The listing builds one solid part. Answer for the finished solid, in the listing's coordinates (mm). Face numbers are marked on the shaded views. A direction names the side the tool comes from. Round coordinates to 2 decimals unless told otherwise and drop trailing zeros. Loops run counter-clockwise (first coordinate to the right, second up) from the corner with the lowest first, then second, coordinate; pieces in that order, holes last. Notation, with made-up numbers: M -3,-17.75 L 34,-17.75 A7 ccw 34,-5.75 Z; hole C -28.75,-11.75 d7. An arc over 180 degrees is marked long. Answer as a JSON object with one key per item and string values.
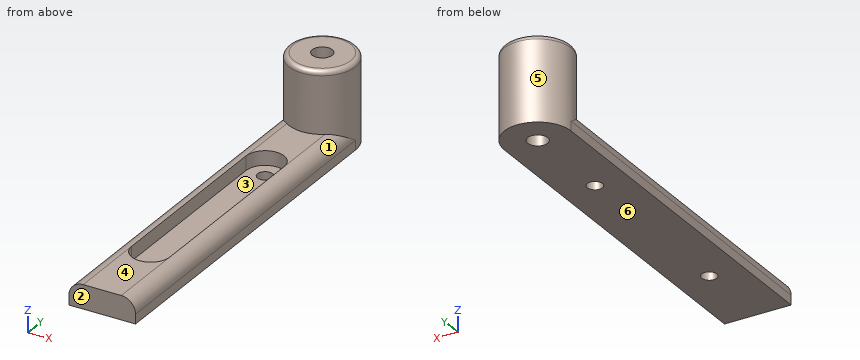
```python
from build123d import *

# Parameters (mm, degrees)
SKETCH1_R           = 7
BOSS_EXTRUDE1_DEPTH = 18
SKETCH2_W           = 14
SKETCH2_H           = 77
BOSS_EXTRUDE2_DEPTH = 5
SKETCH8_R           = 2.1
CUT_EXTRUDE5_DEPTH  = 18
FILLET3_R           = 3
CUT_EXTRUDE6_DEPTH  = 3
SKETCH10_R          = 1.6
CUT_EXTRUDE7_DEPTH  = 3
FILLET4_R           = 1


with BuildPart() as part:
    # Sketch1 → Boss-Extrude1 (new body)
    with BuildSketch(Plane.XY):
        Circle(SKETCH1_R)
    extrude(amount=BOSS_EXTRUDE1_DEPTH)

    # Sketch2 → Boss-Extrude2 (add)
    with BuildSketch(Plane.XY):
        with Locations((0, -38.5)):
            Rectangle(SKETCH2_W, SKETCH2_H)
    extrude(amount=BOSS_EXTRUDE2_DEPTH)

    # Sketch8 → Cut-Extrude5 (cut)
    with BuildSketch(Plane.XY.offset(18)):
        Circle(SKETCH8_R)
    extrude(amount=-CUT_EXTRUDE5_DEPTH, mode=Mode.SUBTRACT)

    # Fillet3
    # the kernel refuses this fillet: 3 mm, written as the material it takes off along each edge
    with BuildSketch(Plane(origin=(7, 7.5, 5), x_dir=(-1, 0, 0), z_dir=(0, -1, 0))) as fillet3_piece_1_section:
        with BuildLine():
            CenterArc((FILLET3_R, FILLET3_R), FILLET3_R, 180, 90)
            Line((0, FILLET3_R), (0, 0))
            Line((0, 0), (FILLET3_R, 0))
        make_face()
    fillet3_piece_1 = extrude(amount=92, mode=Mode.PRIVATE)
    fillet3_piece_1 = fillet3_piece_1 - Plane(origin=(0, 0, 4.306838987), x_dir=(1, 0, 0), z_dir=(0, 0, -1)) * Cylinder(7, 196, mode=Mode.PRIVATE)
    add(fillet3_piece_1, mode=Mode.SUBTRACT)
    with BuildSketch(Plane(origin=(-7, -84.5, 5), x_dir=(0, 0, -1), z_dir=(0, 1, 0))) as fillet3_piece_2_section:
        with BuildLine():
            CenterArc((FILLET3_R, -FILLET3_R), FILLET3_R, 90, 90)
            Line((0, -FILLET3_R), (0, 0))
            Line((0, 0), (FILLET3_R, 0))
        make_face()
    fillet3_piece_2 = extrude(amount=92, mode=Mode.PRIVATE)
    fillet3_piece_2 = fillet3_piece_2 - Plane(origin=(0, 0, 4.306838506), x_dir=(1, 0, 0), z_dir=(0, 0, -1)) * Cylinder(7, 196, mode=Mode.PRIVATE)
    add(fillet3_piece_2, mode=Mode.SUBTRACT)

    # Sketch6 → Cut-Extrude6 (cut)
    with BuildSketch(Plane.XY.offset(5)):
        with BuildLine():
            Line((4, -20), (4, -60))
            ThreePointArc((4, -60), (0, -64), (-4, -60))
            Line((-4, -60), (-4, -20))
            ThreePointArc((-4, -20), (0, -16), (4, -20))
        make_face()
    extrude(amount=-CUT_EXTRUDE6_DEPTH, mode=Mode.SUBTRACT)

    # Sketch10 → Cut-Extrude7 (cut)
    with BuildSketch(Plane.XY.offset(2)):
        with Locations((0, -20)):
            Circle(SKETCH10_R)
        with Locations((0, -60)):
            Circle(SKETCH10_R)
    extrude(amount=-CUT_EXTRUDE7_DEPTH, mode=Mode.SUBTRACT)

    # Fillet4
    fillet4_edges = [part.edges().sort_by_distance(p)[0] for p in [
        (-7, 0, 18),
    ]]
    fillet(fillet4_edges, radius=FILLET4_R)


solid = part.part
```
Item 1: The part is cut by section A-A (x = 0). Give the vertices of the cut face in (y, z).
Values follow:
{"outline": "M -77,0 L -61.6,0 L -61.6,2 L -64,2 L -64,5 L -77,5 Z; M -58.4,0 L -21.6,0 L -21.6,2 L -58.4,2 Z; M -18.4,0 L -2.1,0 L -2.1,18 L -6,18 A1 ccw -7,17 L -7,5 L -16,5 L -16,2 L -18.4,2 Z; M 2.1,0 L 7,0 L 7,17 A1 ccw 6,18 L 2.1,18 Z"}
Item 2: Straight lines are drawn through the part: line 1 (Y direction, x = 0, z = 1.1); line 2 (X direction, y = -28.5, z = 4.25); line 3 (X direction, y = -1.5, z = 6). For each, find the intervals that lie inside material, in ascending order.
Values follow:
{"line 1": "-77 to -61.6, -58.4 to -21.6, -18.4 to -2.1, 2.1 to 7", "line 2": "-5.98 to -4, 4 to 5.98", "line 3": "-6.84 to -1.47, 1.47 to 6.84"}
Item 3: The part is cut by section C-C (z = 15). Give the vertices of the cut face in (x, y).
Values follow:
{"outline": "C 0,0 d14; hole C 0,0 d4.2"}
Item 4: Determine the mould class of the marked faces 1, 2 and 3 for opening direction Y: released by +Y, released by -Y, zero draft, split by the parting line, or undercut.
Values follow:
{"face 1": "zero draft", "face 2": "released by -Y", "face 3": "undercut"}
Item 5: Flat-ended cylindrical pins translate along their axes: P1, Ø4, axis at x = 0, y = 0, coming from the +Z side; P2, Ø4, axis at x = -1, y = -44.5, coming from the +Z side; P3, Ø4, axis at x = -1.5, y = -11.5, coming from the +Z side; P4, Ø6, axis at x = -2, z = 2.5, coming from the +Y side. Find the tip coordinate at first contact, or state that the pin passes through.
Values follow:
{"P1": "through", "P2": "z = 2", "P3": "z = 5", "P4": "y = 7"}
Item 6: Which of the six approach directions +Z, -Z, +X, -X, +Y, -Y give full straight-line access (tool end or side, diameter ignored) to the marked faces 4, 5 and 6?
Values follow:
{"face 4": "+Z, +X, -X, -Y", "face 5": "+Z", "face 6": "-Z, +X, -X, +Y, -Y"}
Item 7: The part is cut by section B-B (y = -31). Give the vertices of the cut face in (x, z), then the cut area to 3 significant figures.
Values follow:
{"outline": "M -7,0 L 7,0 L 7,2 A3 ccw 4,5 L 4,2 L -4,2 L -4,5 A3 ccw -7,2 Z", "area": "42.1 mm^2"}
